from build123d import *

# Parameters (mm, degrees)
RESSALTO_EXTRUS_O1_DEPTH      = 5.3
RESSALTO_EXTRUS_O1_DEPTH_BACK = 3.3
ESBO_O1_3_R                   = 13.75
RESSALTO_EXTRUS_O2_DEPTH      = 3.3
FILETE2_R                     = 0.5
ESBO_O2_R                     = 17
ESBO_O2_R_2                   = 13.75
RESSALTO_EXTRUS_O3_DEPTH      = 2


with BuildPart() as part:
    # Esbo_o1 → Ressalto-extrus_o1 (new body, two sides)
    with BuildSketch(Plane(origin=(0, 0, 0), x_dir=(0, 0, -1), z_dir=(1, 0, 0))) as ressalto_extrus_o1_sk:
        with BuildLine():
            ThreePointArc((0.5, -1.414213562), (1.4531398, -0.37200097), (1.118033989, 1))
            Line((1.118033989, 1), (-1.118033989, 1))
            ThreePointArc((-1.118033989, 1), (-1.4531398, -0.37200097), (-0.5, -1.414213562))
            Line((-0.5, -1.414213562), (-0.5, -3.464101615))
            ThreePointArc((-0.5, -3.464101615), (0, 3.5), (0.5, -3.464101615))
            Line((0.5, -3.464101615), (0.5, -1.414213562))
        make_face()
    extrude(amount=RESSALTO_EXTRUS_O1_DEPTH)
    extrude(ressalto_extrus_o1_sk.sketch, amount=-RESSALTO_EXTRUS_O1_DEPTH_BACK)

    # Esbo_o1_3 → Ressalto-extrus_o2 (add, symmetric)
    with BuildSketch(Plane(origin=(0, 0, 0), x_dir=(0, 0, -1), z_dir=(1, 0, 0))):
        Circle(ESBO_O1_3_R)
        with BuildLine():
            ThreePointArc((3.446771953, 0.608081497), (3.031088913, -1.75), (1.196771953, -3.28903282))
            ThreePointArc((1.196771953, -3.28903282), (2.228560776, -3.144612223), (3.229618168, -3.433280857))
            Line((3.229618168, -3.433280857), (6.244929793, -5.410607922))
            ThreePointArc((6.244929793, -5.410607922), (7.143531761, -6.946693722), (6.462297299, -8.590763273))
            ThreePointArc((6.462297299, -8.590763273), (0, -10.75), (-6.462297299, -8.590763273))
            ThreePointArc((-6.462297299, -8.590763273), (-7.143531761, -6.946693722), (-6.244929793, -5.410607922))
            Line((-6.244929793, -5.410607922), (-3.229618168, -3.433280857))
            ThreePointArc((-3.229618168, -3.433280857), (-2.228560776, -3.144612223), (-1.196771953, -3.28903282))
            ThreePointArc((-1.196771953, -3.28903282), (-3.031088913, -1.75), (-3.446771953, 0.608081497))
            ThreePointArc((-3.446771953, 0.608081497), (-3.837594458, -0.357684134), (-4.588117525, -1.08029095))
            Line((-4.588117525, -1.08029095), (-7.808188807, -2.702963885))
            ThreePointArc((-7.808188807, -2.702963885), (-9.742921821, -2.628468224), (-10.707946608, -0.949936544))
            ThreePointArc((-10.707946608, -0.949936544), (-9.309773091, 5.375), (-4.531304125, 9.748322057))
            ThreePointArc((-4.531304125, 9.748322057), (-2.595140656, 9.751851916), (-1.563259014, 8.113571807))
            Line((-1.563259014, 8.113571807), (-1.358499357, 4.513571807))
            ThreePointArc((-1.358499357, 4.513571807), (-1.609033682, 3.502296357), (-2.25, 2.680951324))
            ThreePointArc((-2.25, 2.680951324), (0, 3.5), (2.25, 2.680951324))
            ThreePointArc((2.25, 2.680951324), (1.609033682, 3.502296357), (1.358499357, 4.513571807))
            Line((1.358499357, 4.513571807), (1.563259014, 8.113571807))
            ThreePointArc((1.563259014, 8.113571807), (2.595140656, 9.751851916), (4.531304125, 9.748322057))
            ThreePointArc((4.531304125, 9.748322057), (9.396801436, 5.221362156), (10.670967882, -1.301131991))
            ThreePointArc((10.670967882, -1.301131991), (9.587779116, -2.713133117), (7.808188807, -2.702963885))
            Line((7.808188807, -2.702963885), (4.588117525, -1.08029095))
            ThreePointArc((4.588117525, -1.08029095), (3.837594458, -0.357684134), (3.446771953, 0.608081497))
        make_face(mode=Mode.SUBTRACT)
    extrude(amount=RESSALTO_EXTRUS_O2_DEPTH, both=True)

    # Filete2
    filete2_edges = [part.edges().sort_by_distance(p)[0] for p in [
        (5.3, 3.5, 0),
    ]]
    fillet(filete2_edges, radius=FILETE2_R)

    # Esbo_o2 → Ressalto-extrus_o3 (add, symmetric)
    with BuildSketch(Plane(origin=(0, 0, 0), x_dir=(0, 0, -1), z_dir=(1, 0, 0))):
        Circle(ESBO_O2_R)
        Circle(ESBO_O2_R_2, mode=Mode.SUBTRACT)
    extrude(amount=RESSALTO_EXTRUS_O3_DEPTH, both=True)


solid = part.part
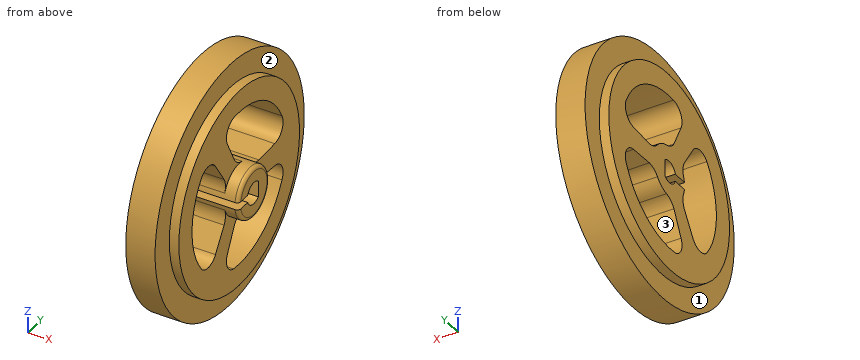
Model file for the job. Use its own axes, mm. Face numbers are marked on the shaded views. A direction names the side the tool comes from. Give positions to 0.01 mm unless a question says otherwise; leave off trailing zeros. Write each loop counter-clockwise with the first axis right and the second up, starting at its lowest first coordinate (ties: lowest second). Pieces come first, ordered by that corner, then holes. Notation, with made-up numbers: (-34, 4) -> (-25, 4) arc R24 ccw to (-25, 23) -> close; hole circle Ø8 at (18.25, -6). An arc over 180 degrees is marked (long way). Write item = value, one per line.
(1) Slice it at A-A, the plane z = 0. Give the cut face in (x, y), then the cut area to 3 significant figures.
Determined:
outline = (-3.3, -13.75) -> (-2, -13.75) -> (-2, -17) -> (2, -17) -> (2, -13.75) -> (3.3, -13.75) -> (3.3, -10.75) -> (-3.3, -10.75) -> close; (-3.3, 1) -> (5.3, 1) -> (5.3, 3) arc R0.5 ccw to (4.8, 3.5) -> (3.3, 3.5) -> (3.3, 13.75) -> (2, 13.75) -> (2, 17) -> (-2, 17) -> (-2, 13.75) -> (-3.3, 13.75) -> close
area = 135 mm2
(2) Slice it at D-D, the plane y = 11. Give the cut face in (x, z), then the cut area to 3 significant figures.
Determined:
outline = (-3.3, -8.25) -> (-2, -8.25) -> (-2, -12.96) -> (2, -12.96) -> (2, -8.25) -> (3.3, -8.25) -> (3.3, 8.25) -> (2, 8.25) -> (2, 12.96) -> (-2, 12.96) -> (-2, 8.25) -> (-3.3, 8.25) -> close
area = 147 mm2
(3) Probe line 1 along Z through (x, y) = (1.25, 5); line 2 along Y through (x, z) = (1.5, -6); line 3 along Y through (x, z) = (4.75, 0). List the from-to ranges inside material, lowest first.
Determined:
line_1 = -16.25 to -9.52, -1.39 to 1.39, 9.52 to 16.25
line_2 = -15.91 to -8.92, -5.25 to -1.79, 8.92 to 15.91
line_3 = 1 to 3.5
(4) Slice it at C-C, the plane x = 1.5. Give the number of separate pieces and of enclosed holes in the cut face, then the cut area to 3 significant figures.
Determined:
separate_pieces = 1
enclosed_holes = 3
area = 652 mm2
(5) Tool access for the marked faces 1, 2 and 3: list every direction of +Z, -Z, +X, -X, +Y, -Y with a clear straight run to the whole face (end or side of a thin tool).
Determined:
face_1 = -X
face_2 = +X
face_3 = +X, -X
(6) Flat gauge pins, fed straight in: P1, Ø5, axis at x = -1, z = 8.5, coming from the -Y side; P2, Ø6, axis at y = 13.5, z = -9, coming from the -X side; P3, Ø5, axis at x = 2, z = -7.5, coming from the +Y side; P4, Ø1.6, axis at x = 2.5, y = -3, coming from the +Z side. Where does each tip first touch, or does it go through?
Determined:
P1 = -15.91
P2 = -3.3
P3 = 16.25
P4 = 16.83
(7) Slice it at B-B, the plane y = -6.5. Give the cut face in (x, z), then the cut area to 3 significant figures.
Determined:
outline = (-3.3, -12.12) -> (-2, -12.12) -> (-2, -15.71) -> (2, -15.71) -> (2, -12.12) -> (3.3, -12.12) -> (3.3, -7.06) -> (-3.3, -7.06) -> close; (-3.3, 7.06) -> (3.3, 7.06) -> (3.3, 12.12) -> (2, 12.12) -> (2, 15.71) -> (-2, 15.71) -> (-2, 12.12) -> (-3.3, 12.12) -> close
area = 95.5 mm2
